Check sheet for the modelled part. Datum: model origin and axes. Units: mm. Round coordinates to 2 decimals unless told otherwise and drop trailing zeros. Loops run counter-clockwise (first coordinate to the right, second up) from the corner with the lowest first, then second, coordinate; pieces in that order, holes last. Notation, with made-up numbers: (46, -6) -> (90, -6) arc R17 ccw to (90, 4) -> close; hole circle Ø8 at (18.25, 22). An arc over 180 degrees is marked (long way). One line per question, with ' | ' between items.
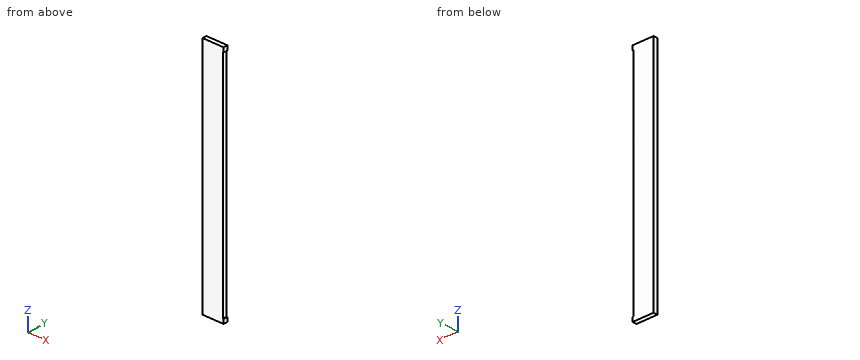
Autodesk Inventor part; units mm, degrees
ref_plane "YZ Plane" through (0, 0, 0) normal (1, 0, 0) x (0, 1, 0)
ref_plane "XZ Plane" through (0, 0, 0) normal (0, 1, 0) x (-1, 0, 0)
ref_plane "XY Plane" through (0, 0, 0) normal (0, 0, 1) x (1, 0, 0)
sketch "Sketch1" plane through (0, 0, 0) normal (0, 1, 0) x (-1, 0, 0)
  line L0 (5, 37) -> (-5, 37)
  line L1 (-5, 37) -> (-5, -37)
  line L2 (-5, -37) -> (5, -37)
  line L3 (5, -37) -> (5, 37)
  point P0 (0, 0)
  dimension "d0" = 10
  dimension "d1" = 74
  dimension "d2" = 5
  dimension "d3" = 37
extrude "Extrusion1" add sketch "Sketch1" along normal blind 2
sketch "Sketch2" plane through (5, 0, 37) normal (1, 0, 0) x (0, 0, -1)
  line L0 (74, 2) -> (0, 2)
  line L1 (74, 0) -> (0, 0)
  line L2 (0, 2) -> (2, 2)
  line L3 (2, 2) -> (2, 0)
  line L4 (2, 0) -> (0, 0)
  line L5 (0, 0) -> (0, 2)
  line L6 (2, 0) -> (74, 0)
  line L7 (74, 0) -> (74, 2)
  line L8 (74, 2) -> (2, 2)
  line L9 (2, 2) -> (2, 0)
  line L10 (74, 0) -> (72, 0)
  line L11 (72, 0) -> (72, 2)
  line L12 (72, 2) -> (74, 2)
  line L13 (74, 2) -> (74, 0)
  point P0 (37, 0)
  point P1 (2, 2)
  dimension "d6" = 72
extrude "Extrusion2" cut sketch "Sketch2" against normal blind 0.3 contours L11 L1 L3 L0
sketch "Sketch3" plane through (5, 0, -37) normal (0, 0, -1) x (-1, 0, 0)
  line L0 (10, 0) -> (10, 2)
  line L1 (0, 0) -> (0, 2)
  line L2 (10, 0) -> (0, 0)
  line L3 (0, 0) -> (0, 2)
  line L4 (0, 2) -> (10, 2)
  line L5 (10, 2) -> (10, 0)
  point P0 (5, 0)
extrude "Extrusion3" add sketch "Sketch3" along normal blind 36
sketch "Sketch4" plane through (0, 2, 0) normal (0, 1, 0) x (1, 0, 0)
  line L0 (-5, 73) -> (5, 73)
  line L1 (4.7, -35) -> (4.7, 35)
  line L2 (5, 73) -> (4.7, 73)
  line L3 (4.7, 73) -> (4.7, 35)
  line L4 (4.7, 35) -> (5, 35)
  line L5 (5, 35) -> (5, 73)
  line L6 (5, 35) -> (5, 73)
  line L7 (5, 73) -> (4.7, 73)
  line L8 (4.7, 73) -> (4.7, 71)
  line L9 (4.7, 71) -> (5, 71)
  line L10 (5, 71) -> (5, 73)
  line L11 (4.7, 71) -> (4.6, 71)
  line L12 (4.6, 71) -> (4.6, -35)
  line L13 (4.6, -35) -> (4.7, -35)
  line L14 (4.7, -35) -> (4.7, 71)
  point P0 (0, 0)
  dimension "d11" = 0.1
extrude "Extrusion4" cut sketch "Sketch4" against normal blind 18.25 contours L9 L5 L4 L3 | L3 L1 L13 L12 L11
sketch "Sketch5" plane through (0, 2, 0) normal (0, 1, 0) x (1, 0, 0)
  point P0 (0, 0)
equation "\"BendRadius\" = Thickness"
equation "\"BendReliefWidth\" = Thickness"
equation "\"BendReliefDepth\" = 0.5 * Thickness"
equation "\"CornerReliefSize\" = 4 * Thickness"
equation "\"MinimumRemnant\" = 2 * Thickness"
equation "\"TransitionRadius\" = BendRadius"
equation "\"JacobiRadiusSize\" = BendRadius"
equation "\"GapSize\" = Thickness"
properties part number "modelGateCover"
(1) Sectioned sample at B-B, the plane z = 2. Record the cut outline in (x, y).
Answer:
outline: (-5, 0) -> (4.6, 0) -> (4.6, 2) -> (-5, 2) -> close
(2) Go/stop test with flat-tipped pins: pin 1 (0.6 mm diameter, centred on y = 0.5, z = -8.5, fed in from +X); pin 2 (6 mm diameter, centred on x = 3.5, z = 5.5, fed in from -Y). Record where each tip stops, or that it passes through.
Answer:
pin 1: stops at x = 4.6 | pin 2: stops at y = 0
(3) Scan line: probe 1 along X at (y, z) = (1.3, 12). Record every from-to range of solid material in increasing order.
Answer:
probe 1: x = -5 to 4.6
(4) Sectioned sample at A-A, the plane y = 1.5. Record the cut outline in (x, z), and give its area (3 significant figures).
Answer:
outline: (-5, -73) -> (5, -73) -> (5, -71) -> (4.6, -71) -> (4.6, 35) -> (5, 35) -> (5, 37) -> (-5, 37) -> close | area: 1,060 mm2
